Geometry check sheet. Reference: drawing and pictorial views, mm from the part's lowest x, y, z. Coordinates: 2 decimals unless noted, no trailing zeros. Loops run counter-clockwise (first coordinate to the right, second up) from the corner with the lowest first, then second, coordinate; pieces in that order, holes last. Notation, with made-up numbers: (37.25, 7.5) -> (55.25, 7.5) arc R30 cw to (55.25, 36.5) -> close; hole circle Ø10 at (18.5, 57). An arc over 180 degrees is marked (long way). Answer as a JSON object with one key per item and string values.
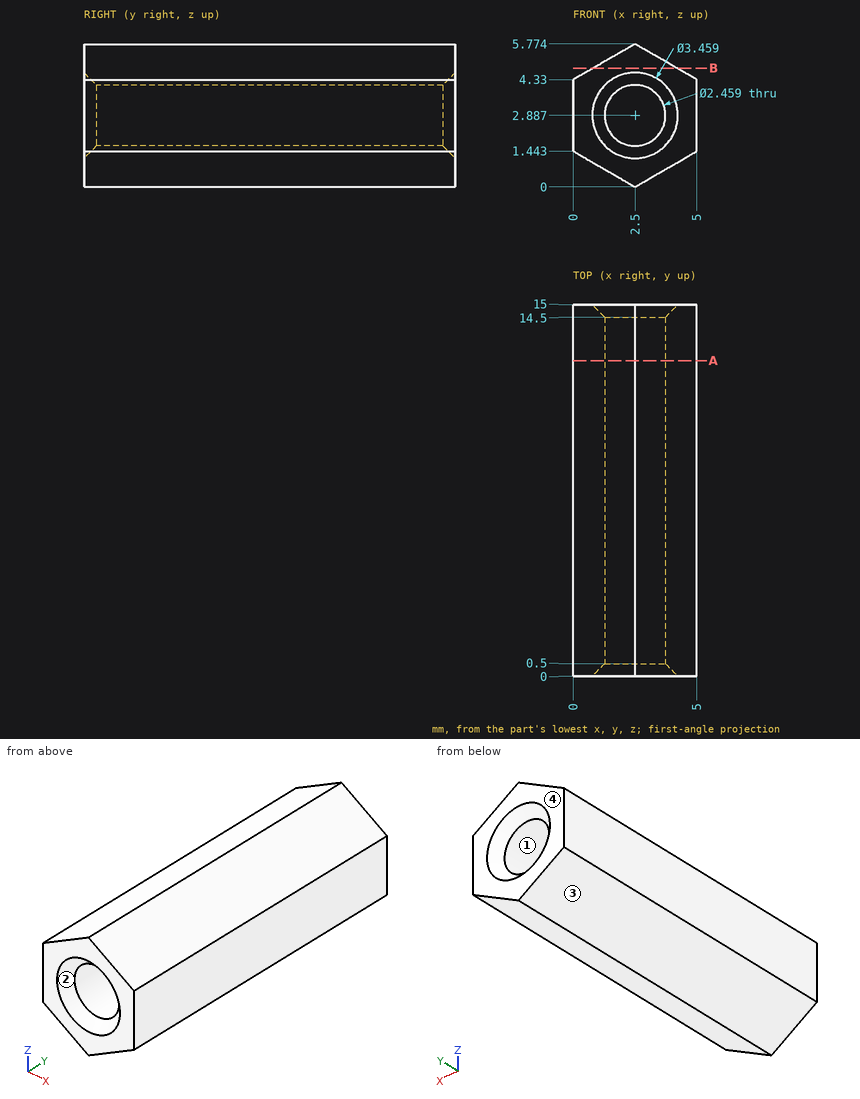
1. Section check B-B, the plane z = 4.8. Record the boundary of the cut face in (x, y).
Evaluation:
{"outline": "(0.81, 0) -> (4.19, 0) -> (4.19, 15) -> (0.81, 15) -> close"}
2. Mould release check, pull along Z, two halves, no side actions. Record for the marked faces 1, 2, 3 and 4: released by +Z, released by -Z, zero draft, split by the parting line, or undercut.
Evaluation:
{"face 1": "undercut", "face 2": "undercut", "face 3": "released by -Z", "face 4": "zero draft"}
3. Thickness scan on probe 1 along X at (y, z) = (4.25, 3.2); probe 2 along X at (y, z) = (11.5, 2.45); probe 3 along Z at (x, y) = (3.3, 4) (1 decimal). Record the ranges inside material, lowest first. Write a range as from..to.
Evaluation:
{"probe 1": "x = 0..1.31, 3.69..5", "probe 2": "x = 0..1.35, 3.65..5", "probe 3": "z = 0.5..2, 3.8..5.3"}
4. Section check A-A, the plane y = 12.75. Record the boundary of the cut face in (x, z), then the cut area to 3 significant figures.
Evaluation:
{"outline": "(0, 1.44) -> (2.5, 0) -> (5, 1.44) -> (5, 4.33) -> (2.5, 5.77) -> (0, 4.33) -> close; hole circle Ø2.46 at (2.5, 2.89)", "area": "16.9 mm^2"}
5. Depth check by flat-ended pin: P1, Ø3, axis at x = 3.5, y = 12, coming from the -Z side. Enter the tip coordinate at first touch or a pass-through.
Evaluation:
{"P1": "stops at z = 0"}
